Geometry check sheet. Reference: the model listing, model coordinates, mm. Face numbers are marked on the shaded views. A direction names the side the tool comes from. Round coordinates to 2 decimals unless told otherwise and drop trailing zeros. Write each loop counter-clockwise with the first axis right and the second up, starting at its lowest first coordinate (ties: lowest second). Pieces come first, ordered by that corner, then holes. Notation, with made-up numbers: (34, -6) -> (85, -6) arc R28 cw to (85, 27) -> close; hole circle Ø1 at (48.25, 11.25). An arc over 180 degrees is marked (long way). One line per question, with ' | ' between items.
```python
from build123d import *

# Parameters (mm, degrees)
F0_W      = 25.4
F0_H      = 50.8
F1_DEPTH  = 25.4
F2_R      = 8.635626
F3_DEPTH  = 24.638
F3_FACE_R = 8.635626
F4_DEPTH  = 36.322
F5_W      = 21.968006
F5_H      = 18.33639
F6_DEPTH  = 0.4826


with BuildPart() as f1:
    # F0 (on Front) → F1 (new body)
    with BuildSketch(Plane.XZ):
        Rectangle(F0_W, F0_H)
    extrude(amount=F1_DEPTH)

    # F2 (on face) → F3 (cut)
    with BuildSketch(Plane.XZ.offset(25.4)):
        Circle(F2_R)
    extrude(amount=-F3_DEPTH, mode=Mode.SUBTRACT)

    # F3_face (on face) → F4 (join)
    with BuildSketch(Plane.XZ.offset(0.762)):
        Circle(F3_FACE_R)
    extrude(amount=F4_DEPTH)

    # F5 (on face) → F6 (join)
    with BuildSketch(Plane.XZ.offset(37.084)):
        Rectangle(F5_W, F5_H)
    extrude(amount=F6_DEPTH)


solid = f1.part
```
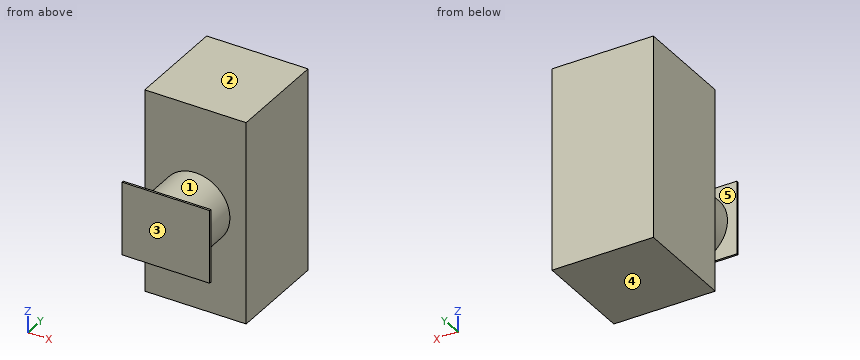
(1) Draft check along Y on the marked faces 1, 2 and 3. Enter one of: +Y half, -Y half, draft (parallel to the pull), parting line (faces both ways), or undercut.
Resolved:
face 1: undercut | face 2: draft | face 3: -Y half
(2) Sectioned sample at A-A on z = 0. Record the cut outline in (x, y).
Resolved:
outline: (-12.7, -25.4) -> (-8.64, -25.4) -> (-8.64, -37.08) -> (-10.98, -37.08) -> (-10.98, -37.57) -> (10.98, -37.57) -> (10.98, -37.08) -> (8.64, -37.08) -> (8.64, -25.4) -> (12.7, -25.4) -> (12.7, 0) -> (-12.7, 0) -> close
(3) Sectioned sample at D-D on z = 10. Record the cut outline in (x, y).
Resolved:
outline: (-12.7, -25.4) -> (12.7, -25.4) -> (12.7, 0) -> (-12.7, 0) -> close
(4) Sectioned sample at B-B on x = 0. Record the cut outline in (y, z).
Resolved:
outline: (-37.57, -9.17) -> (-37.08, -9.17) -> (-37.08, -8.64) -> (-25.4, -8.64) -> (-25.4, -25.4) -> (0, -25.4) -> (0, 25.4) -> (-25.4, 25.4) -> (-25.4, 8.64) -> (-37.08, 8.64) -> (-37.08, 9.17) -> (-37.57, 9.17) -> close
(5) Go/stop test with flat-tipped pins: pin 1 (8 mm diameter, centred on y = -29.5, z = 10, fed in from +X); pin 2 (10 mm diameter, centred on x = -1, z = -16.5, fed in from -Y); pin 3 (14.5 mm diameter, centred on x = 3, z = -1.5, fed in from +Y); pin 4 (10 mm diameter, centred on x = 4, y = -30.5, fed in from -Z). Record where each tip stops, or that it passes through.
Resolved:
pin 1: stops at x = 6.21 | pin 2: stops at y = -25.4 | pin 3: stops at y = 0 | pin 4: stops at z = -8.64
(6) Sectioned sample at C-C on y = -28. Record the cut outline in (x, z), then the cut area to 3 significant figures.
Resolved:
outline: circle Ø17.27 at (0, 0) | area: 234 mm2
(7) Material ranges on line 1 (Y direction, x = -9.5, z = -6.5); line 2 (Y direction, x = -2.25, z = -21.5); line 3 (Z direction, x = 3, y = -29), recorded low to high.
Resolved:
line 1: y = -37.57 to -37.08, -25.4 to 0 | line 2: y = -25.4 to 0 | line 3: z = -8.1 to 8.1
(8) Access from +Z, -Z, +X, -X, +Y, -Y to the whole of each face (thin tool, end or side, straight path). Record for the marked faces 4 and 5.
Resolved:
face 4: -Z, +X, -X, +Y, -Y | face 5: none
